Geometry check sheet. Reference: the model listing, model coordinates, mm. A direction names the side the tool comes from. Round coordinates to 2 decimals unless told otherwise and drop trailing zeros. Loops run counter-clockwise (first coordinate to the right, second up) from the corner with the lowest first, then second, coordinate; pieces in that order, holes last. Notation, with made-up numbers: (75, 50) - (134, 50) arc R13 cw to (134, 71) - close; hole circle Ø6 at (16.25, -18). An arc over 180 degrees is marked (long way). Answer in a Markdown table with one row per item. Add a question column.
```python
from build123d import *


with BuildPart() as f2:
    # F2: sweep along a path in F1
    with BuildLine(Plane.YZ) as f2_path:
        ThreePointArc((0, 0), (128.283823392, -77.0044991359), (189.3310906342, -213.6048775888))
        ThreePointArc((189.3310906342, -213.6048775888), (257.8411517666, -346.8010377561), (397.1464335918, -401.836335659))
    # F0 (on Front) → F2 (sweep)
    with BuildSketch(Plane.XZ):
        Polygon((76.2, 74.93), (-76.2, 74.93), (-76.2, 38.1), (-19.05, 38.1), (-19.05, -38.1), (-76.2, -38.1), (-76.2, -74.93), (76.2, -74.93), (76.2, -38.1), (19.05, -38.1), (19.05, 38.1), (76.2, 38.1), align=None)
    sweep(path=f2_path.line)


solid = f2.part
```
Q1. Scan lines: line 1 (X direction, y = 189.5, z = -134); line 2 (Y direction, x = 31.5, z = -102); line 3 (Z direction, x = -24.5, y = 74). Record each from-to range of solid material in increasing order. Write a range as from..to.
Q2. Cross-section at A-A, the plane x = 52.5. Enter the section's corners in (y, z), plus the area to 3 significant figures.
Q3. Set-up check for faces 5 (the cylindrical face through (-48.025, 105.31, -106.834)), 6 (the cylindrical face through (48.03, 274.87, -312.11)), 7 (the flat face through (76.2, 164, -288)): record each of +Z, -Z, +X, -X, +Y, -Y from which the full face is reachable in a straight line by a thin tool's end or side.
Q4. Release check for a two-part mould opening along Z. For faces 1 (the flat face through (76.2, 213, -125)), 2 (the cylindrical face through (1.07, 219.65, -410.73)), 3 (the cylindrical face through (47.225, 105.31, -106.834)), 4 (the cylindrical face through (48.03, 148.42, -44)) record: +Z half, -Z half, draft (parallel to the pull), parting line (faces both ways), or undercut.
Q5. Cross-section at B-B, the plane z = -260. Enter the section's corners in (x, y).
Q6. Cross-section at C-C, the plane x = -2.5. Enter the section's corners in (y, z), plus the area to 3 significant figures.
Q7. Cross-section at D-D, the plane y = 30. Enter the section's corners in (x, z).
Q8. Depth check by flat-ended pin: P1, Ø4, axis at x = 25.5, y = 359.5, coming from the -Z side; P2, Ø4, axis at x = -32.5, z = -232.5, coming from the -Y side; P3, Ø8, axis at x = 0.5, z = -331.5, coming from the +Y side. Enter the tip coordinate at first touch or a pass-through.
Check sheet entries:
| question | item | result |
|---|---|---|
| 1 | line 1 | -19.05..19.05 |
| 1 | line 2 | 50.04..101.18, 191.46..232.21 |
| 1 | line 3 | -124.3..-76.14, 11.74..51.89 |
| 2 | outline | (0, -74.93) arc R177.17 cw to (118.97, -239.37) arc R286.13 ccw to (413.44, -474.97) - (405.43, -439.03) arc R249.95 cw to (153.55, -226.7) arc R212.3 ccw to (0, -38.1) - close; (0, 38.1) arc R286.35 cw to (225.11, -200.51) arc R175.92 ccw to (388.86, -364.65) - (380.86, -328.7) arc R140.97 cw to (259.69, -187.84) arc R322.5 ccw to (0, 74.93) - close |
| 2 | area | 43,700 mm² |
| 3 | face 5 | -X |
| 3 | face 6 | +X |
| 3 | face 7 | +Z, -Z, +X, +Y, -Y |
| 4 | face 1 | draft |
| 4 | face 2 | -Z half |
| 4 | face 3 | undercut |
| 4 | face 4 | undercut |
| 5 | outline | (-76.2, 123.44) - (76.2, 123.44) - (76.2, 160.97) - (19.05, 160.97) - (19.05, 239.65) - (76.2, 239.65) - (76.2, 278.8) - (-76.2, 278.8) - (-76.2, 239.65) - (-19.05, 239.65) - (-19.05, 160.97) - (-76.2, 160.97) - close |
| 6 | outline | (0, -74.93) arc R177.17 cw to (118.97, -239.37) arc R286.13 ccw to (413.44, -474.97) - (380.86, -328.7) arc R140.97 cw to (259.69, -187.84) arc R322.5 ccw to (0, 74.93) - close |
| 6 | area | 88,900 mm² |
| 7 | outline | (-76.2, -88.61) - (76.2, -88.61) - (76.2, -49.15) - (19.05, -49.15) - (19.05, 30.16) - (76.2, 30.16) - (76.2, 67.93) - (-76.2, 67.93) - (-76.2, 30.16) - (-19.05, 30.16) - (-19.05, -49.15) - (-76.2, -49.15) - close |
| 8 | P1 | z = -472.57 |
| 8 | P2 | y = 118.6 |
| 8 | P3 | y = 382.37 |
